```python
from build123d import *

# Parameters (mm, degrees)
SKETCH1_R           = 20.5
SKETCH1_R_2         = 19.5
BOSS_EXTRUDE1_DEPTH = 34
SKETCH2_W           = 2.79800491
SKETCH2_H           = 1.698963444
CUT_EXTRUDE1_DEPTH  = 35


with BuildPart() as part:
    # Sketch1 → Boss-Extrude1 (new body)
    with BuildSketch(Plane.XY):
        Circle(SKETCH1_R)
        Circle(SKETCH1_R_2, mode=Mode.SUBTRACT)
    extrude(amount=BOSS_EXTRUDE1_DEPTH)

    # Sketch2 → Cut-Extrude1 (cut, through all)
    with BuildSketch(Plane.XY.offset(34)):
        with Locations((0.015441627, 20.064895184)):
            Rectangle(SKETCH2_W, SKETCH2_H)
    extrude(amount=-CUT_EXTRUDE1_DEPTH, mode=Mode.SUBTRACT)


solid = part.part
```
Here's how the part is built. I have some questions about the finished solid (model axes, mm). Coordinates: 2 decimals unless noted, no trailing zeros. Loops run counter-clockwise (first coordinate to the right, second up) from the corner with the lowest first, then second, coordinate; pieces in that order, holes last. Notation, with made-up numbers: M -2,87.5 L 6,87.5 A23 cw 6,118.5 Z; hole C 68,53.5 d6. An arc over 180 degrees is marked long. One line per item, written item: value.
1. Please list where these lines run through material, in increasing order: probe 1 along X at (y, z) = (0, 18); probe 2 along Y at (x, z) = (-13, 16); probe 3 along Y at (x, z) = (0, 23).
Geometry says:
probe 1: x = -20.5 to -19.5, 19.5 to 20.5
probe 2: y = -15.85 to -14.53, 14.53 to 15.85
probe 3: y = -20.5 to -19.5
2. Imagine slicing it at C-C (z = 10). List the corners of the cut face in (x, y) for me.
Geometry says:
outline: M -1.38,19.45 L -1.38,20.45 A20.5 ccw long 1.41,20.45 L 1.41,19.45 A19.5 cw long Z
3. Imagine slicing it at A-A (y = -11.5). List the corners of the cut face in (x, z) for me.
Geometry says:
outline: M -16.97,0 L -15.75,0 L -15.75,34 L -16.97,34 Z; M 15.75,0 L 16.97,0 L 16.97,34 L 15.75,34 Z
4. Imagine slicing it at B-B (x = 18). List the corners of the cut face in (y, z) for me, and give its area (3 significant figures).
Geometry says:
outline: M -9.81,0 L -7.5,0 L -7.5,34 L -9.81,34 Z; M 7.5,0 L 9.81,0 L 9.81,34 L 7.5,34 Z
area: 157 mm2
5. Imagine slicing it at D-D (x = 0). List the corners of the cut face in (y, z) for me, and give its area (3 significant figures).
Geometry says:
outline: M -20.5,0 L -19.5,0 L -19.5,34 L -20.5,34 Z
area: 34.0 mm2
6. Will these pins go through, and if not, where does the flat tip stop? pin 1 Ø3 at (x, z) = (-4, 29) entering from +Y; pin 2 Ø3 at (y, z) = (11, 8.5) entering from -X; pin 3 Ø8 at (y, z) = (10.5, 24) entering from -X.
Geometry says:
pin 1: stops at y = 20.35
pin 2: stops at x = -18.17
pin 3: stops at x = -19.44
